Check sheet for the modelled part. Datum: model origin and axes. Units: mm. Face numbers are marked on the shaded views. A direction names the side the tool comes from. Coordinates: 2 decimals unless noted, no trailing zeros. Loops run counter-clockwise (first coordinate to the right, second up) from the corner with the lowest first, then second, coordinate; pieces in that order, holes last.
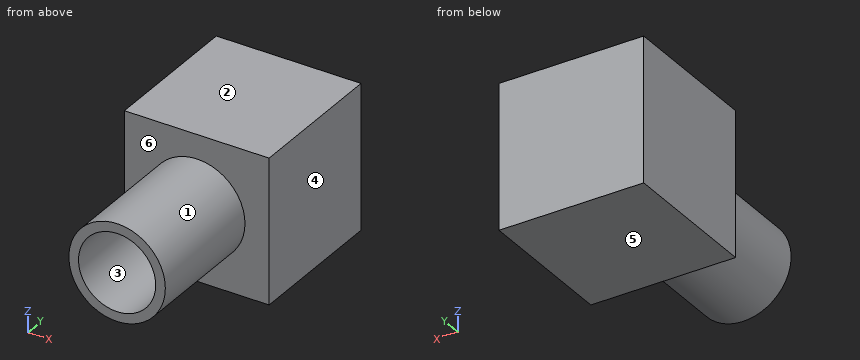
```python
from build123d import *

# Parameters (mm, degrees)
F0_W     = 150
F0_H     = 150
F1_DEPTH = 150
F3_R     = 50
F4_DEPTH = 130
F5_R     = 40
F6_DEPTH = 125


with BuildPart() as f1:
    # F0 (on Top) → F1 (new body)
    with BuildSketch(Plane.XY):
        Rectangle(F0_W, F0_H)
    extrude(amount=F1_DEPTH)

    # F3 (on face) → F4 (join)
    with BuildSketch(Plane.XZ.offset(75)):
        with Locations((0, 75)):
            Circle(F3_R)
    extrude(amount=F4_DEPTH)

    # F5 (on face) → F6 (cut)
    with BuildSketch(Plane.XZ.offset(205)):
        with Locations((0, 75)):
            Circle(F5_R)
    extrude(amount=-F6_DEPTH, mode=Mode.SUBTRACT)


solid = f1.part
```
1) Section check A-A on x = 0. Enter the section's corners in (y, z), plus the area to 3 significant figures.
Answer sheet:
outline: (-205, 25) - (-75, 25) - (-75, 0) - (75, 0) - (75, 150) - (-75, 150) - (-75, 125) - (-205, 125) - (-205, 115) - (-80, 115) - (-80, 35) - (-205, 35) - close
area: 25,500 mm2
2) Set-up check for the marked faces 5 and 6: record each of +Z, -Z, +X, -X, +Y, -Y from which the full face is reachable in a straight line by a thin tool's end or side.
Answer sheet:
face 5: -Z, +X, -X, +Y, -Y
face 6: -Y
3) Section check B-B on z = 75. Enter the section's corners in (x, y), plus the area to 3 significant figures.
Answer sheet:
outline: (-75, -75) - (-50, -75) - (-50, -205) - (-40, -205) - (-40, -80) - (40, -80) - (40, -205) - (50, -205) - (50, -75) - (75, -75) - (75, 75) - (-75, 75) - close
area: 25,500 mm2
4) Mould release check, pull along X, two halves, no side actions. Record for the marked faces 1, 2, 3 and 4: +X half, -X half, draft (parallel to the pull), parting line (faces both ways), or undercut.
Answer sheet:
face 1: parting line
face 2: draft
face 3: undercut
face 4: +X half
5) Section check D-D on z = 139.5. Enter the section's corners in (x, y).
Answer sheet:
outline: (-75, -75) - (75, -75) - (75, 75) - (-75, 75) - close
6) Scan lines: line 1 (Z direction, x = 0, y = -122); line 2 (Y direction, x = 62.5, z = 35); line 3 (Y direction, x = -2.5, z = 98). Record each from-to range of solid material in increasing order.
Answer sheet:
line 1: z = 25 to 35, 115 to 125
line 2: y = -75 to 75
line 3: y = -80 to 75
7) Depth check by flat-ended pin: pin 1 (10 mm diameter, centred on x = 47, y = -107, fed in from +Z); pin 2 (10 mm diameter, centred on x = -9, y = 3, fed in from -Z); pin 3 (2 mm diameter, centred on x = -16, y = -82.5, fed in from -Z). Enter the tip coordinate at first touch or a pass-through.
Answer sheet:
pin 1: stops at z = 102.13
pin 2: stops at z = 0
pin 3: stops at z = 27.3
8) Section check C-C on y = -137. Enter the section's corners in (x, z).
Answer sheet:
outline: circle Ø100 at (0, 75); hole circle Ø80 at (0, 75)
